Check sheet for the modelled part. Datum: model origin and axes. Units: mm. A direction names the side the tool comes from. Round coordinates to 2 decimals unless told otherwise and drop trailing zeros. Write each loop counter-clockwise with the first axis right and the second up, starting at its lowest first coordinate (ties: lowest second). Pieces come first, ordered by that corner, then holes. Notation, with made-up numbers: (64, 45) -> (95, 45) arc R31 ccw to (95, 73) -> close; hole circle Ø7 at (77.5, 32.5). An arc over 180 degrees is marked (long way). Put each result on its own line as item: value. Start each with the question number.
from build123d import *

# Parameters (mm, degrees)
SKETCH2_R           = 3.75
BOSS_EXTRUDE1_DEPTH = 6.5
SKETCH3_R           = 5
BOSS_EXTRUDE2_DEPTH = 2
SKETCH4_R           = 1.25
CUT_EXTRUDE1_DEPTH  = 6.5
SKETCH5_R           = 2.75
CUT_EXTRUDE2_DEPTH  = 5


with BuildPart() as part:
    # Sketch2 → Boss-Extrude1 (new body)
    with BuildSketch(Plane(origin=(0, 0, 0), x_dir=(1, 0, 0), z_dir=(0, 1, 0))):
        Circle(SKETCH2_R)
    extrude(amount=BOSS_EXTRUDE1_DEPTH)

    # Sketch3 → Boss-Extrude2 (add)
    with BuildSketch(Plane(origin=(0, 6.5, 0), x_dir=(1, 0, 0), z_dir=(0, 1, 0))):
        Circle(SKETCH3_R)
    extrude(amount=BOSS_EXTRUDE2_DEPTH)

    # Sketch4 → Cut-Extrude1 (cut)
    with BuildSketch(Plane.XZ):
        Circle(SKETCH4_R)
    extrude(amount=-CUT_EXTRUDE1_DEPTH, mode=Mode.SUBTRACT)

    # Sketch5 → Cut-Extrude2 (cut)
    with BuildSketch(Plane(origin=(0, 8.5, 0), x_dir=(1, 0, 0), z_dir=(0, 1, 0))):
        Circle(SKETCH5_R)
    extrude(amount=-CUT_EXTRUDE2_DEPTH, mode=Mode.SUBTRACT)


solid = part.part
1. Section check C-C, the plane y = 5.75. Enter the section's corners in (x, z), then the cut area to 3 significant figures.
2. Access from +Z, -Z, +X, -X, +Y, -Y to the whole of each face (thin tool, end or side, straight path). Record for faces 1 (the cylindrical face through (-3.746, 3.204, -0.165)), 2 (the cylindrical face through (-0.596, 6.035, 2.685)), 3 (the cylindrical face through (-1.08, 7.49, 4.88)).
3. Section check B-B, the plane x = 0. Enter the section's corners in (y, z), then the cut area to 3 significant figures.
4. Section check D-D, the plane x = 2.25. Enter the section's corners in (y, z).
5. Material ranges on L1, parallel to X at y = 7.4, z = 0; L2, parallel to Z at x = 0, y = 1.1; L3, parallel to Z at x = 0, y = 5.5, recorded low to high. Write a range as [from, to].
6. Section check A-A, the plane z = 0. Enter the section's corners in (x, y), then the cut area to 3 significant figures.
7. Gauge pin test, flat ends, axial feed: P1, Ø3, axis at y = 4.5, z = 3.5, coming from the -X side; P2, Ø5, axis at x = 3.5, y = 5, coming from the -Z side; P3, Ø1, axis at y = 2.5, z = 3, coming from the -X side. Record the tip position at first contact, or that the pin passes through.
Reply:
1. outline: circle Ø7.5 at (0, 0); hole circle Ø5.5 at (0, 0)
1. area: 20.4 mm2
2. face 1: -Y
2. face 2: +Y
2. face 3: +Y, -Y
3. outline: (0, -3.75) -> (6.5, -3.75) -> (6.5, -5) -> (8.5, -5) -> (8.5, -2.75) -> (3.5, -2.75) -> (3.5, -1.25) -> (0, -1.25) -> close; (0, 1.25) -> (3.5, 1.25) -> (3.5, 2.75) -> (8.5, 2.75) -> (8.5, 5) -> (6.5, 5) -> (6.5, 3.75) -> (0, 3.75) -> close
3. area: 32.5 mm2
4. outline: (0, -3) -> (6.5, -3) -> (6.5, -4.47) -> (8.5, -4.47) -> (8.5, -1.58) -> (3.5, -1.58) -> (3.5, 1.58) -> (8.5, 1.58) -> (8.5, 4.47) -> (6.5, 4.47) -> (6.5, 3) -> (0, 3) -> close
5. L1: x = [-5, -2.75], [2.75, 5]
5. L2: z = [-3.75, -1.25], [1.25, 3.75]
5. L3: z = [-3.75, -2.75], [2.75, 3.75]
6. outline: (-5, 6.5) -> (-3.75, 6.5) -> (-3.75, 0) -> (-1.25, 0) -> (-1.25, 3.5) -> (-2.75, 3.5) -> (-2.75, 8.5) -> (-5, 8.5) -> close; (1.25, 0) -> (3.75, 0) -> (3.75, 6.5) -> (5, 6.5) -> (5, 8.5) -> (2.75, 8.5) -> (2.75, 3.5) -> (1.25, 3.5) -> close
6. area: 32.5 mm2
7. P1: stops at x = -3.17
7. P2: stops at z = -4.77
7. P3: stops at x = -2.8
